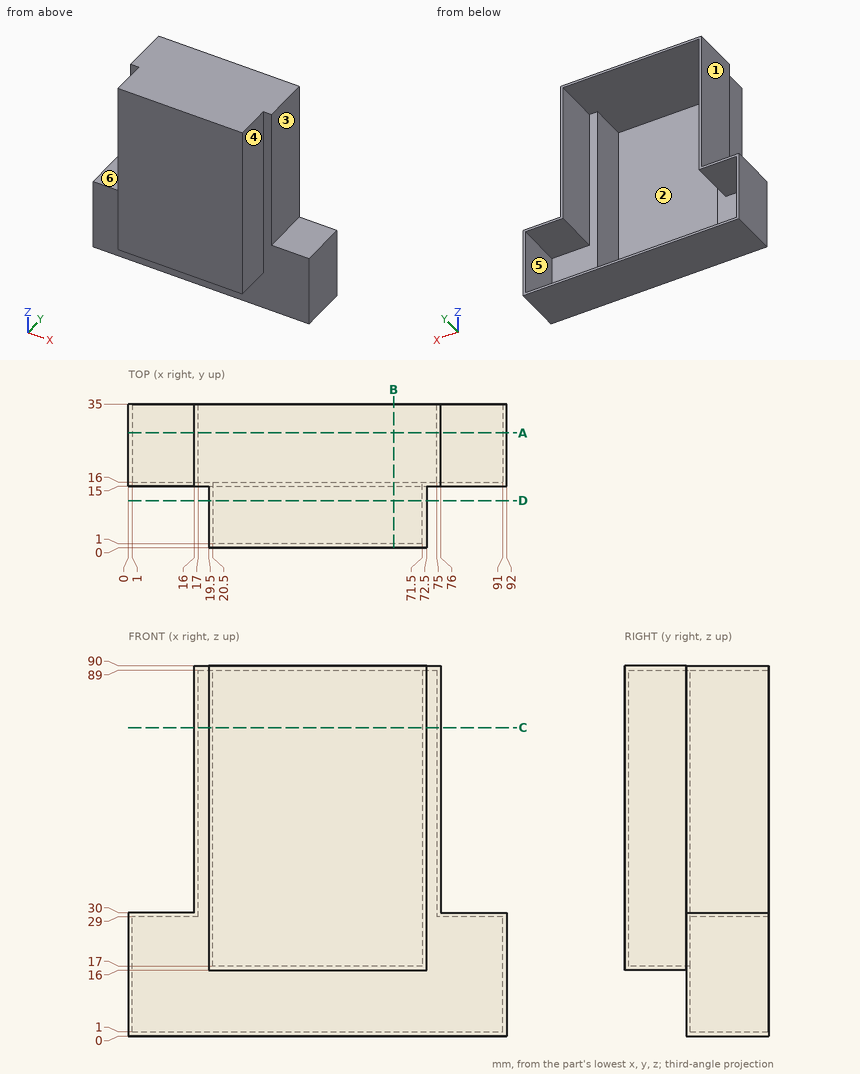
Geometry: see drawing. Coordinates: mm, zero at the bounding-box minimum. A direction names the side the tool comes from. Round coordinates to 2 decimals unless told otherwise and drop trailing zeros. Loops run counter-clockwise (first coordinate to the right, second up) from the corner with the lowest first, then second, coordinate; pieces in that order, holes last.
(1) Contact query for flat-ended pins moving along their axis: pin 1 Ø8 at (x, y) = (5, 23.5) entering from -Z; pin 2 Ø5 at (x, y) = (81.5, 24) entering from +Z; pin 3 Ø3 at (y, z) = (3.5, 53) entering from +X; pin 4 Ø16.5 at (y, z) = (7, 56.5) entering from +X. Output: stop coordinate, or through.
From the geometry:
pin 1: stops at z = 0
pin 2: stops at z = 30
pin 3: stops at x = 72.5
pin 4: stops at x = 76
(2) Access query for the marked faces 1, 2 and 3. Directions: +Z, -Z, +X, -X, +Y, -Y. A direction counts if a zero-diameter tool reaches every point of the face in a straight line with its end or side. Return the directions, or none.
From the geometry:
face 1: +Z, -X, +Y, -Y
face 2: +Y
face 3: +Z, +X, +Y, -Y
(3) Material intervals for probe 1 along Z at (x, y) = (70, 28); probe 2 along Z at (x, y) = (49, 2); probe 3 along X at (y, z) = (16.5, 35.5), sorted ascending.
From the geometry:
probe 1: z = 0 to 1, 89 to 90
probe 2: z = 16 to 17, 89 to 90
probe 3: x = 16 to 17, 75 to 76
(4) Section query C-C (z = 75). Output: boundary loops of the cut face in (x, y), and give its area (3 significant figures).
From the geometry:
outline: (16, 15) - (19.5, 15) - (19.5, 0) - (72.5, 0) - (72.5, 15) - (76, 15) - (76, 35) - (75, 35) - (75, 16) - (71.5, 16) - (71.5, 1) - (20.5, 1) - (20.5, 16) - (17, 16) - (17, 35) - (16, 35) - close
area: 128 mm2
(5) Pull-direction query (X, two-part tool) for the marked faces 4, 5 and 6; classes: +X half, -X half, draft (parallel to the pull), parting line (faces both ways), or undercut.
From the geometry:
face 4: +X half
face 5: undercut
face 6: draft
(6) Section query B-B (x = 64.5). Output: boundary loops of the cut face in (y, z).
From the geometry:
outline: (0, 16) - (15, 16) - (15, 0) - (35, 0) - (35, 1) - (16, 1) - (16, 17) - (1, 17) - (1, 89) - (35, 89) - (35, 90) - (0, 90) - close
(7) Section query D-D (y = 11.5). Output: boundary loops of the cut face in (x, z).
From the geometry:
outline: (19.5, 16) - (72.5, 16) - (72.5, 90) - (19.5, 90) - close; hole (20.5, 17) - (71.5, 17) - (71.5, 89) - (20.5, 89) - close
(8) Section query A-A (y = 28). Output: boundary loops of the cut face in (x, z).
From the geometry:
outline: (0, 0) - (92, 0) - (92, 30) - (76, 30) - (76, 90) - (16, 90) - (16, 30) - (0, 30) - close; hole (1, 1) - (91, 1) - (91, 29) - (75, 29) - (75, 89) - (17, 89) - (17, 29) - (1, 29) - close
